from build123d import *

# Parameters (mm, degrees)
F0_R     = 5.522275
F0_R_2   = 1.27325
F1_DEPTH = 1.3716
F2_DEPTH = 7.6962
F3_DEPTH = 9.652
F4_DEPTH = 10.668


with BuildPart() as f1:
    # F0 (on Top) → F1 (new body)
    with BuildSketch(Plane.XY):
        Circle(F0_R)
        Circle(F0_R_2, mode=Mode.SUBTRACT)
    extrude(amount=F1_DEPTH)

    # F0 (on Top) → F2 (join)
    with BuildSketch(Plane.XY):
        with BuildLine():
            ThreePointArc((7.517685, -1.599688), (7.678957, -0.700082), (7.732966, 0.212269))
            ThreePointArc((7.732966, 0.212269), (6.299561, 4.697166), (2.530744, 7.519396))
            ThreePointArc((2.530744, 7.519396), (1.706006, 7.754703), (0.860282, 7.897234))
            ThreePointArc((0.860282, 7.897234), (0.43081, 7.933226), (0, 7.945235))
            ThreePointArc((0, 7.945235), (-0.456383, 7.931756), (-0.911175, 7.891366))
            ThreePointArc((-0.911175, 7.891366), (-0.921549, 7.890128), (-0.93192, 7.888876))
            ThreePointArc((-0.93192, 7.888876), (-1.746141, 7.745513), (-2.540403, 7.516043))
            ThreePointArc((-2.540403, 7.516043), (-6.71147, 4.053485), (-7.584297, -1.296775))
            ThreePointArc((-7.584297, -1.296775), (-7.3792, -2.099913), (-7.089314, -2.876483))
            ThreePointArc((-7.089314, -2.876483), (-6.673834, -3.693971), (-6.164503, -4.456529))
            ThreePointArc((-6.164503, -4.456529), (-5.619672, -5.099798), (-5.008058, -5.67994))
            ThreePointArc((-5.008058, -5.67994), (-0.155544, -7.519133), (4.767017, -5.8766))
            ThreePointArc((4.767017, -5.8766), (5.40017, -5.322795), (5.969425, -4.703495))
            ThreePointArc((5.969425, -4.703495), (6.511698, -3.958649), (6.961536, -3.154597))
            ThreePointArc((6.961536, -3.154597), (7.281236, -2.392031), (7.517685, -1.599688))
        make_face()
        Circle(F0_R, mode=Mode.SUBTRACT)
    extrude(amount=F2_DEPTH)

    # F0 (on Top) → F3 (join)
    with BuildSketch(Plane.XY):
        with BuildLine():
            ThreePointArc((7.517685, -1.599688), (7.678957, -0.700082), (7.732966, 0.212269))
            ThreePointArc((7.732966, 0.212269), (6.299561, 4.697166), (2.530744, 7.519396))
            ThreePointArc((2.530744, 7.519396), (1.706006, 7.754703), (0.860282, 7.897234))
            ThreePointArc((0.860282, 7.897234), (0.43081, 7.933226), (0, 7.945235))
            ThreePointArc((0, 7.945235), (-0.456383, 7.931756), (-0.911175, 7.891366))
            ThreePointArc((-0.911175, 7.891366), (-0.921549, 7.890128), (-0.93192, 7.888876))
            ThreePointArc((-0.93192, 7.888876), (-1.746141, 7.745513), (-2.540403, 7.516043))
            ThreePointArc((-2.540403, 7.516043), (-6.71147, 4.053485), (-7.584297, -1.296775))
            ThreePointArc((-7.584297, -1.296775), (-7.3792, -2.099913), (-7.089314, -2.876483))
            ThreePointArc((-7.089314, -2.876483), (-6.673834, -3.693971), (-6.164503, -4.456529))
            ThreePointArc((-6.164503, -4.456529), (-5.619672, -5.099798), (-5.008058, -5.67994))
            ThreePointArc((-5.008058, -5.67994), (-0.155544, -7.519133), (4.767017, -5.8766))
            ThreePointArc((4.767017, -5.8766), (5.40017, -5.322795), (5.969425, -4.703495))
            ThreePointArc((5.969425, -4.703495), (6.511698, -3.958649), (6.961536, -3.154597))
            ThreePointArc((6.961536, -3.154597), (7.281236, -2.392031), (7.517685, -1.599688))
        make_face()
        Circle(F0_R, mode=Mode.SUBTRACT)
        with BuildLine():
            ThreePointArc((0.860282, 7.897234), (1.706006, 7.754703), (2.530744, 7.519396))
            Line((2.530744, 7.519396), (2.530744, 13.906265))
            Line((2.530744, 13.906265), (0.914411, 13.906265))
            Line((0.914411, 13.906265), (0.860282, 7.897234))
        make_face()
        with BuildLine():
            Line((12.93451, -4.900329), (7.517685, -1.599688))
            ThreePointArc((7.517685, -1.599688), (7.281236, -2.392031), (6.961536, -3.154597))
            Line((6.961536, -3.154597), (12.093005, -6.28136))
            Line((12.093005, -6.28136), (12.93451, -4.900329))
        make_face()
        with BuildLine():
            Line((11.13613, -7.851729), (5.969425, -4.703495))
            ThreePointArc((5.969425, -4.703495), (5.40017, -5.322795), (4.767017, -5.8766))
            Line((4.767017, -5.8766), (10.2893, -9.241499))
            Line((10.2893, -9.241499), (11.13613, -7.851729))
        make_face()
        with BuildLine():
            ThreePointArc((-0.93192, 7.888876), (-0.921549, 7.890128), (-0.911175, 7.891366))
            Line((-0.911175, 7.891366), (-0.911175, 13.906265))
            Line((-0.911175, 13.906265), (-2.540403, 13.906265))
            Line((-2.540403, 13.906265), (-2.540403, 7.516043))
            ThreePointArc((-2.540403, 7.516043), (-1.746141, 7.745513), (-0.93192, 7.888876))
        make_face()
        with BuildLine():
            Line((-10.655986, -8.807297), (-5.008058, -5.67994))
            ThreePointArc((-5.008058, -5.67994), (-5.619672, -5.099798), (-6.164503, -4.456529))
            Line((-6.164503, -4.456529), (-11.445815, -7.380884))
            Line((-11.445815, -7.380884), (-10.655986, -8.807297))
        make_face()
        with BuildLine():
            ThreePointArc((-7.089314, -2.876483), (-7.3792, -2.099913), (-7.584297, -1.296775))
            Line((-7.584297, -1.296775), (-13.11972, -4.357855))
            Line((-13.11972, -4.357855), (-12.332427, -5.779687))
            Line((-12.332427, -5.779687), (-7.089314, -2.876483))
        make_face()
    extrude(amount=F3_DEPTH)

    # F0 (on Top) → F4 (join)
    with BuildSketch(Plane.XY):
        with BuildLine():
            ThreePointArc((7.517685, -1.599688), (7.678957, -0.700082), (7.732966, 0.212269))
            ThreePointArc((7.732966, 0.212269), (6.299561, 4.697166), (2.530744, 7.519396))
            ThreePointArc((2.530744, 7.519396), (1.706006, 7.754703), (0.860282, 7.897234))
            ThreePointArc((0.860282, 7.897234), (0.43081, 7.933226), (0, 7.945235))
            ThreePointArc((0, 7.945235), (-0.456383, 7.931756), (-0.911175, 7.891366))
            ThreePointArc((-0.911175, 7.891366), (-0.921549, 7.890128), (-0.93192, 7.888876))
            ThreePointArc((-0.93192, 7.888876), (-1.746141, 7.745513), (-2.540403, 7.516043))
            ThreePointArc((-2.540403, 7.516043), (-6.71147, 4.053485), (-7.584297, -1.296775))
            ThreePointArc((-7.584297, -1.296775), (-7.3792, -2.099913), (-7.089314, -2.876483))
            ThreePointArc((-7.089314, -2.876483), (-6.673834, -3.693971), (-6.164503, -4.456529))
            ThreePointArc((-6.164503, -4.456529), (-5.619672, -5.099798), (-5.008058, -5.67994))
            ThreePointArc((-5.008058, -5.67994), (-0.155544, -7.519133), (4.767017, -5.8766))
            ThreePointArc((4.767017, -5.8766), (5.40017, -5.322795), (5.969425, -4.703495))
            ThreePointArc((5.969425, -4.703495), (6.511698, -3.958649), (6.961536, -3.154597))
            ThreePointArc((6.961536, -3.154597), (7.281236, -2.392031), (7.517685, -1.599688))
        make_face()
        Circle(F0_R, mode=Mode.SUBTRACT)
        with BuildLine():
            ThreePointArc((0.860282, 7.897234), (1.706006, 7.754703), (2.530744, 7.519396))
            Line((2.530744, 7.519396), (2.530744, 13.906265))
            Line((2.530744, 13.906265), (0.914411, 13.906265))
            Line((0.914411, 13.906265), (0.860282, 7.897234))
        make_face()
        with BuildLine():
            Line((12.93451, -4.900329), (7.517685, -1.599688))
            ThreePointArc((7.517685, -1.599688), (7.281236, -2.392031), (6.961536, -3.154597))
            Line((6.961536, -3.154597), (12.093005, -6.28136))
            Line((12.093005, -6.28136), (12.93451, -4.900329))
        make_face()
        with BuildLine():
            Line((11.13613, -7.851729), (5.969425, -4.703495))
            ThreePointArc((5.969425, -4.703495), (5.40017, -5.322795), (4.767017, -5.8766))
            Line((4.767017, -5.8766), (10.2893, -9.241499))
            Line((10.2893, -9.241499), (11.13613, -7.851729))
        make_face()
        with BuildLine():
            ThreePointArc((-0.93192, 7.888876), (-0.921549, 7.890128), (-0.911175, 7.891366))
            Line((-0.911175, 7.891366), (-0.911175, 13.906265))
            Line((-0.911175, 13.906265), (-2.540403, 13.906265))
            Line((-2.540403, 13.906265), (-2.540403, 7.516043))
            ThreePointArc((-2.540403, 7.516043), (-1.746141, 7.745513), (-0.93192, 7.888876))
        make_face()
        with BuildLine():
            Line((-10.655986, -8.807297), (-5.008058, -5.67994))
            ThreePointArc((-5.008058, -5.67994), (-5.619672, -5.099798), (-6.164503, -4.456529))
            Line((-6.164503, -4.456529), (-11.445815, -7.380884))
            Line((-11.445815, -7.380884), (-10.655986, -8.807297))
        make_face()
        with BuildLine():
            ThreePointArc((-7.089314, -2.876483), (-7.3792, -2.099913), (-7.584297, -1.296775))
            Line((-7.584297, -1.296775), (-13.11972, -4.357855))
            Line((-13.11972, -4.357855), (-12.332427, -5.779687))
            Line((-12.332427, -5.779687), (-7.089314, -2.876483))
        make_face()
    extrude(amount=F4_DEPTH)


solid = f1.part
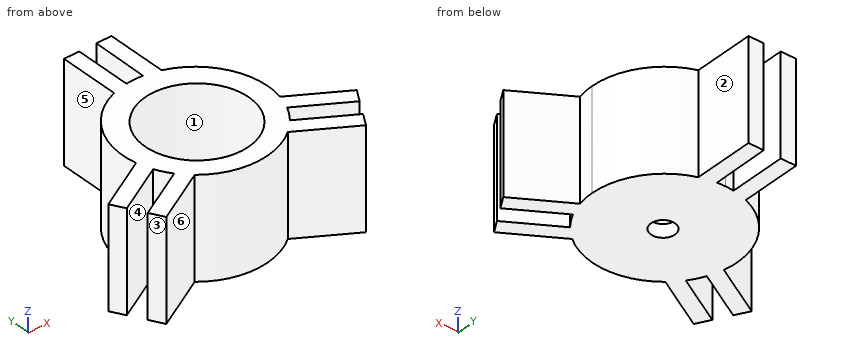
Could you check a few things on this model? Use its own coordinates, in mm. Face numbers are marked on the shaded views. A direction names the side the tool comes from. Coordinates: 2 decimals unless noted, no trailing zeros. Write each loop counter-clockwise with the first axis right and the second up, starting at its lowest first coordinate (ties: lowest second). Pieces come first, ordered by that corner, then holes. Notation, with made-up numbers: (-19, 42) - (-12, 42) arc R18 cw to (-12, 50) - close; hole circle Ø3 at (35, -25.75). An arc over 180 degrees is marked (long way). Put each result on its own line as item: value. Start each with the question number.
Q1. Which directions (+Z, -Z, +X, -X, +Y, -Y) give clear straight access to the entire face, cutting with the end or side of a thin tool? Please do the marked faces 4, 5 and 6.
Q2. I'm going to push flat-ended pins straight in: P1, Ø1.8, axis at y = 12, z = 6.5, coming from the +X side; P2, Ø1.5, axis at y = -6, z = 1.5, coming from the +X side; P3, Ø8, axis at x = 0, y = 0.5, coming from the -Z side; P4, Ø5.5, axis at x = 0, y = 0.5, coming from the +Z side. Where does each tip first touch, or does it pass through?
Q3. I want a section at B-B on z = 9.25. Write out the boundary of the cut face in (x, y).
Q4. Thinking about a two-plate mould opening in Y: for the marked faces 1, 2 and 3, which applies, pulls with the +Y half, pulls with the -Y half, needs draft (parallel to the pull), parting line crosses it, or undercut?
Q5. Please list where these lines run through material, in increasing order: L1, parallel to X at y = 8.5, z = 4.75; L2, parallel to Z at x = -3, y = -0.5; L3, parallel to Y at x = -1.5, z = 1.5.
Q6. I want a section at C-C on x = -3.75. Write out the boundary of the cut face in (y, z).
Q7. I want a section at A-A on x = 9.75. Write out the boundary of the cut face in (y, z), plus the area to 3 significant figures.
Checks:
1. face 4: +Z, -Z
1. face 5: +Z, -Z, -X, +Y
1. face 6: +Z, -Z, -Y
2. P1: x = 2.53
2. P2: x = 12.72
2. P3: z = 0
2. P4: z = 1.37
3. outline: (-13.12, -4.36) - (-12.33, -5.78) - (-7.09, -2.88) arc R7.73 ccw to (-6.16, -4.46) - (-11.45, -7.38) - (-10.66, -8.81) - (-5.01, -5.68) arc R7.73 ccw to (4.77, -5.88) - (10.29, -9.24) - (11.14, -7.85) - (5.97, -4.7) arc R7.73 ccw to (6.96, -3.15) - (12.09, -6.28) - (12.93, -4.9) - (7.52, -1.6) arc R7.73 ccw to (7.73, 0.21) arc R7.73 ccw to (2.53, 7.52) - (2.53, 13.91) - (0.91, 13.91) - (0.86, 7.9) arc R7.73 ccw to (0, 7.95) arc R7.73 ccw to (-0.91, 7.89) - (-0.91, 13.91) - (-2.54, 13.91) - (-2.54, 7.52) arc R7.73 ccw to (-7.58, -1.3) - close; hole circle Ø11.04 at (0, 0)
4. face 1: undercut
4. face 2: needs draft
4. face 3: pulls with the -Y half
5. L1: -2.54 to -0.91, 0.87 to 2.53
5. L2: 0 to 1.37
5. L3: -7.37 to -5.31, 5.31 to 13.91
6. outline: (-6.55, 0) - (6.98, 0) - (6.98, 10.67) - (4.05, 10.67) - (4.05, 1.37) - (-4.05, 1.37) - (-4.05, 10.67) - (-6.55, 10.67) - close
7. outline: (-8.91, 0) - (-7.01, 0) - (-7.01, 10.67) - (-8.91, 10.67) - close; (-4.85, 0) - (-2.96, 0) - (-2.96, 10.67) - (-4.85, 10.67) - close
7. area: 40.5 mm²
